Read the model definition and answer for the solid it produces. Units are mm, in the model's axes. Give positions to 0.01 mm unless a question says otherwise; leave off trailing zeros. Loops run counter-clockwise (first coordinate to the right, second up) from the corner with the lowest first, then second, coordinate; pieces in that order, holes last. Notation, with made-up numbers: (53, 43) -> (110, 43) arc R18 cw to (110, 56) -> close; hole circle Ø5 at (73.25, 26). An arc over 180 degrees is marked (long way). Answer as CSV lines item,"result". Start each with the question number.
```python
from build123d import *

# Parameters (mm, degrees)
F0_W     = 177.8
F0_H     = 254
F0_R     = 15
F0_R_2   = 20
F0_R_3   = 10
F0_R_4   = 45
F1_DEPTH = 6.35


with BuildPart() as f1:
    # F0 (on Top) → F1 (new body)
    with BuildSketch(Plane.XY):
        Rectangle(F0_W, F0_H)
        with Locations((-60, -75)):
            Circle(F0_R, mode=Mode.SUBTRACT)
        with Locations((0, -75)):
            Circle(F0_R_2, mode=Mode.SUBTRACT)
        with Locations((60, -75)):
            Circle(F0_R, mode=Mode.SUBTRACT)
        with Locations((-60, 0)):
            Circle(F0_R_3, mode=Mode.SUBTRACT)
        with Locations((-60, 75)):
            Circle(F0_R, mode=Mode.SUBTRACT)
        Circle(F0_R_4, mode=Mode.SUBTRACT)
        with Locations((60, 0)):
            Circle(F0_R_3, mode=Mode.SUBTRACT)
        with Locations((0, 75)):
            Circle(F0_R_2, mode=Mode.SUBTRACT)
        with Locations((60, 75)):
            Circle(F0_R, mode=Mode.SUBTRACT)
    extrude(amount=F1_DEPTH)


solid = f1.part
```
(1) Find the intervals of material crossed by line 1 along Y through (x, z) = (-60, 4); line 2 along Y through (x, z) = (0, 2); line 3 along X through (y, z) = (1, 1.75), in increasing order. Write a range as from..to.
(2) The mould has two halves that part along Y. Classify faces 1 (the face through (-88.9, -2, 3)), 2 (the face through (-63.252, -89.643, 3.131)), 3 (the face through (-1, 127, 3)): pulls with the +Y half, pulls with the -Y half, needs draft (parallel to the pull), parting line crosses it, or undercut.
(3) Find section C-C on z = 3.25. Give the number of separate pieces and of enclosed holes in the cut face, then the cut area to 3 significant figures.
(4) This flat-tipped pin is pushed along its axis until it touches: P1, Ø18, axis at x = -60, y = -75, coming from the +Z side. Where does it stop, or does it pass through?
(5) Find section B-B on y = -75. Write down the section's boundary in (x, z).
(6) Find section A-A on x = -60. Write down the section's boundary in (y, z).
(7) Find section D-D on y = -28.5. Write down the section's boundary in (x, z), then the cut area to 3 significant figures.
Answer block:
1,line 1,"y = -127..-90, -60..-10, 10..60, 90..127"
1,line 2,"y = -127..-95, -55..-45, 45..55, 95..127"
1,line 3,"x = -88.9..-69.95, -50.05..-44.99, 44.99..50.05, 69.95..88.9"
2,face 1,"needs draft"
2,face 2,"undercut"
2,face 3,"pulls with the +Y half"
3,separate pieces,"1"
3,enclosed holes,"9"
3,area,"32,800 mm2"
4,P1,"passes through"
5,outline,"(-88.9, 0) -> (-75, 0) -> (-75, 6.35) -> (-88.9, 6.35) -> close; (-45, 0) -> (-20, 0) -> (-20, 6.35) -> (-45, 6.35) -> close; (20, 0) -> (45, 0) -> (45, 6.35) -> (20, 6.35) -> close; (75, 0) -> (88.9, 0) -> (88.9, 6.35) -> (75, 6.35) -> close"
6,outline,"(-127, 0) -> (-90, 0) -> (-90, 6.35) -> (-127, 6.35) -> close; (-60, 0) -> (-10, 0) -> (-10, 6.35) -> (-60, 6.35) -> close; (10, 0) -> (60, 0) -> (60, 6.35) -> (10, 6.35) -> close; (90, 0) -> (127, 0) -> (127, 6.35) -> (90, 6.35) -> close"
7,outline,"(-88.9, 0) -> (-34.82, 0) -> (-34.82, 6.35) -> (-88.9, 6.35) -> close; (34.82, 0) -> (88.9, 0) -> (88.9, 6.35) -> (34.82, 6.35) -> close"
7,area,"687 mm2"
